```python
from build123d import *
from build123d.topology import SkipClean

# Parameters (mm, degrees)
SKETCH1_R           = 7.5
BOSS_EXTRUDE1_DEPTH = 19
SKETCH1_3_R         = 10
SKETCH1_3_R_2       = 7.5
CUT_EXTRUDE1_DEPTH  = 13
SKETCH2_R           = 6
SKETCH2_R_2         = 5
BOSS_EXTRUDE3_DEPTH = 18
SKETCH11_R          = 10
SKETCH11_R_2        = 7.5
BOSS_EXTRUDE4_DEPTH = 13
SKETCH12_R          = 10
CUT_EXTRUDE7_DEPTH  = 13
SKETCH3_W           = 60
SKETCH3_H           = 5
CUT_EXTRUDE2_DEPTH  = 180
SKETCH4_R           = 7.5
CUT_EXTRUDE3_DEPTH  = 8
SKETCH5_R           = 9
CUT_EXTRUDE4_DEPTH  = 130
SKETCH6_R           = 11
CUT_EXTRUDE5_DEPTH  = 15
SKETCH7_R           = 10
CUT_EXTRUDE6_DEPTH  = 15


with BuildPart() as part:
    # Sketch1 → Boss-Extrude1 (new body)
    with BuildSketch(Plane(origin=(0, 0, 0), x_dir=(1, 0, 0), z_dir=(0, 1, 0))):
        with BuildLine():
            Line((15, 0), (165, 0))
            ThreePointArc((165, 0), (175.606601718, 4.393398282), (180, 15))
            Line((180, 15), (180, 105))
            ThreePointArc((180, 105), (175.606601718, 115.606601718), (165, 120))
            Line((165, 120), (15, 120))
            ThreePointArc((15, 120), (4.393398282, 115.606601718), (0, 105))
            Line((0, 105), (0, 15))
            ThreePointArc((0, 15), (4.393398282, 4.393398282), (15, 0))
        make_face()
        with Locations(Location((15, 15, 0), (0, 0, 270))):
            Circle(SKETCH1_R, mode=Mode.SUBTRACT)
        with Locations(Location((15, 105, 0), (0, 0, 270))):
            Circle(SKETCH1_R, mode=Mode.SUBTRACT)
        with Locations(Location((165, 105, 0), (0, 0, 270))):
            Circle(SKETCH1_R, mode=Mode.SUBTRACT)
        with Locations(Location((165, 15, 0), (0, 0, 270))):
            Circle(SKETCH1_R, mode=Mode.SUBTRACT)
    extrude(amount=BOSS_EXTRUDE1_DEPTH)

    # Sketch1_3 → Cut-Extrude1 (cut)
    # profile 1 of 4: a face of its own
    with BuildSketch(Plane(origin=(0, 0, 0), x_dir=(1, 0, 0), z_dir=(0, 1, 0))):
        with Locations(Location((165, 105, 0), (0, 0, 90))):
            Circle(SKETCH1_3_R)
        with Locations(Location((165, 105, 0), (0, 0, 270))):
            Circle(SKETCH1_3_R_2, mode=Mode.SUBTRACT)
    # profile 2 of 4: a face of its own
    with BuildSketch(Plane(origin=(0, 0, 0), x_dir=(1, 0, 0), z_dir=(0, 1, 0))):
        with Locations(Location((165, 15, 0), (0, 0, 90))):
            Circle(SKETCH1_3_R)
        with Locations(Location((165, 15, 0), (0, 0, 270))):
            Circle(SKETCH1_3_R_2, mode=Mode.SUBTRACT)
    # profile 3 of 4: a face of its own
    with BuildSketch(Plane(origin=(0, 0, 0), x_dir=(1, 0, 0), z_dir=(0, 1, 0))):
        with Locations(Location((15, 105, 0), (0, 0, 90))):
            Circle(SKETCH1_3_R)
        with Locations(Location((15, 105, 0), (0, 0, 270))):
            Circle(SKETCH1_3_R_2, mode=Mode.SUBTRACT)
    # profile 4 of 4: a face of its own
    with BuildSketch(Plane(origin=(0, 0, 0), x_dir=(1, 0, 0), z_dir=(0, 1, 0))):
        with Locations(Location((15, 15, 0), (0, 0, 90))):
            Circle(SKETCH1_3_R)
        with Locations(Location((15, 15, 0), (0, 0, 270))):
            Circle(SKETCH1_3_R_2, mode=Mode.SUBTRACT)
    extrude(amount=CUT_EXTRUDE1_DEPTH, mode=Mode.SUBTRACT)

    # Sketch2 → Boss-Extrude3 (add, symmetric)
    with BuildSketch(Plane.XY.offset(-60)):
        with BuildLine():
            Line((25, 0), (155, 0))
            Line((155, 0), (155, 168))
            ThreePointArc((155, 168), (90, 233), (25, 168))
            Line((25, 168), (25, 0))
        make_face()
        with Locations((90, 218)):
            Circle(SKETCH2_R, mode=Mode.SUBTRACT)
        with Locations((140, 168)):
            Circle(SKETCH2_R, mode=Mode.SUBTRACT)
        with Locations((90, 58)):
            Circle(SKETCH2_R, mode=Mode.SUBTRACT)
        with Locations((40, 168)):
            Circle(SKETCH2_R, mode=Mode.SUBTRACT)
        with Locations((40, 108)):
            Circle(SKETCH2_R, mode=Mode.SUBTRACT)
        with Locations((140, 108)):
            Circle(SKETCH2_R, mode=Mode.SUBTRACT)
        with Locations((54.644660941, 72.644660941)):
            Circle(SKETCH2_R_2, mode=Mode.SUBTRACT)
        with Locations((125.355339059, 203.355339059)):
            Circle(SKETCH2_R_2, mode=Mode.SUBTRACT)
        with BuildLine():
            Line((67.460330813, 141.223829382), (67.460330813, 134.776170618))
            ThreePointArc((67.460330813, 134.776170618), (90, 73), (112.539669187, 134.776170618))
            Line((112.539669187, 134.776170618), (112.539669187, 141.223829382))
            ThreePointArc((112.539669187, 141.223829382), (90, 203), (67.460330813, 141.223829382))
        make_face(mode=Mode.SUBTRACT)
    extrude(amount=BOSS_EXTRUDE3_DEPTH, both=True)

    # Sketch11 → Boss-Extrude4 (add)
    # profile 1 of 4: a face of its own
    with SkipClean():  # the faces are left unmerged after this step: merging them gives an invalid solid
        with BuildSketch(Plane.XZ):
            with Locations((15, -15)):
                Circle(SKETCH11_R)
            with Locations(Location((15, -15, 0), (0, 0, 270))):
                Circle(SKETCH11_R_2, mode=Mode.SUBTRACT)
        # profile 2 of 4: a face of its own
        with BuildSketch(Plane.XZ):
            with Locations((165, -15)):
                Circle(SKETCH11_R)
            with Locations(Location((165, -15, 0), (0, 0, 270))):
                Circle(SKETCH11_R_2, mode=Mode.SUBTRACT)
        # profile 3 of 4: a face of its own
        with BuildSketch(Plane.XZ):
            with Locations((165, -105)):
                Circle(SKETCH11_R)
            with Locations(Location((165, -105, 0), (0, 0, 270))):
                Circle(SKETCH11_R_2, mode=Mode.SUBTRACT)
        # profile 4 of 4: a face of its own
        with BuildSketch(Plane.XZ):
            with Locations((15, -105)):
                Circle(SKETCH11_R)
            with Locations(Location((15, -105, 0), (0, 0, 270))):
                Circle(SKETCH11_R_2, mode=Mode.SUBTRACT)
        extrude(amount=-BOSS_EXTRUDE4_DEPTH)

    # Sketch12 → Cut-Extrude7 (cut)
    with BuildSketch(Plane(origin=(0, 19, 0), x_dir=(1, 0, 0), z_dir=(0, 1, 0))):
        with Locations(Location((15, 105, 0), (0, 0, 270))):
            Circle(SKETCH12_R)
        with Locations(Location((165, 105, 0), (0, 0, 270))):
            Circle(SKETCH12_R)
        with Locations(Location((165, 15, 0), (0, 0, 270))):
            Circle(SKETCH12_R)
        with Locations(Location((15, 15, 0), (0, 0, 270))):
            Circle(SKETCH12_R)
    extrude(amount=-CUT_EXTRUDE7_DEPTH, mode=Mode.SUBTRACT)

    # Sketch3 → Cut-Extrude2 (cut)
    with BuildSketch(Plane(origin=(180, 0, 0), x_dir=(0, 0, -1), z_dir=(1, 0, 0))):
        with Locations((60, 2.5)):
            Rectangle(SKETCH3_W, SKETCH3_H)
    extrude(amount=-CUT_EXTRUDE2_DEPTH, mode=Mode.SUBTRACT)

    # Sketch4 → Cut-Extrude3 (cut)
    with BuildSketch(Plane(origin=(0, 0, -78), x_dir=(-1, 0, 0), z_dir=(0, 0, -1))):
        with Locations((-90, 218)):
            Circle(SKETCH4_R)
        with Locations((-40, 168)):
            Circle(SKETCH4_R)
        with Locations((-40, 108)):
            Circle(SKETCH4_R)
        with Locations((-90, 58)):
            Circle(SKETCH4_R)
        with Locations((-140, 108)):
            Circle(SKETCH4_R)
        with Locations((-140, 168)):
            Circle(SKETCH4_R)
    cut_extrude3 = extrude(amount=-CUT_EXTRUDE3_DEPTH, mode=Mode.SUBTRACT)

    # Mirror1: Cut-Extrude3 across plane
    add(cut_extrude3.mirror(Plane.XY.offset(-60)), mode=Mode.SUBTRACT)

    # Sketch5 → Cut-Extrude4 (cut)
    with BuildSketch(Plane.ZY.offset(-25)):
        with Locations((-60, 138)):
            Circle(SKETCH5_R)
    extrude(amount=-CUT_EXTRUDE4_DEPTH, mode=Mode.SUBTRACT)

    # Sketch6 → Cut-Extrude5 (cut)
    with BuildSketch(Plane.ZY.offset(-25)):
        with Locations((-60, 138)):
            Circle(SKETCH6_R)
    extrude(amount=-CUT_EXTRUDE5_DEPTH, mode=Mode.SUBTRACT)

    # Sketch7 → Cut-Extrude6 (cut)
    with BuildSketch(Plane(origin=(155, 0, 0), x_dir=(0, 0, -1), z_dir=(1, 0, 0))):
        with Locations((60, 138)):
            Circle(SKETCH7_R)
    extrude(amount=-CUT_EXTRUDE6_DEPTH, mode=Mode.SUBTRACT)


solid = part.part
```
Input: part model. Units: mm. Frame: model coordinates. A direction names the side the tool comes from. Give positions to 0.01 mm unless a question says otherwise; leave off trailing zeros. Loops run counter-clockwise (first coordinate to the right, second up) from the corner with the lowest first, then second, coordinate; pieces in that order, holes last. Notation, with made-up numbers: (-8, 67.5) -> (36, 67.5) arc R24 cw to (36, 78.5) -> close; hole circle Ø11 at (-32.75, 14.25). An arc over 180 degrees is marked (long way). Use a Markdown table: item, result.
Q1. Access query for faces 1 (the flat face through (88, 224, -50)), 2 (the cylindrical face through (40.976, 175.436, -74.056)), 3 (the cylindrical face through (155.24, 12.59, -17.17)), 4 (the flat face through (112.54, 138, -73)), 5 (the flat face through (91, 5, -60)). Directions: +Z, -Z, +X, -X, +Y, -Y. A direction counts if a zero-diameter tool reaches every point of the face in a straight line with its end or side. Return the directions, or none.
Entries:
| item | result |
|---|---|
| face 1 | +Z |
| face 2 | -Z |
| face 3 | +Y |
| face 4 | +Z, -Z |
| face 5 | +X, -X, -Y |
Q2. Section query A-A, the plane y = 58. Return the cut outline in (x, z).
Entries:
| item | result |
|---|---|
| outline | (25, -78) -> (82.5, -78) -> (82.5, -70) -> (84, -70) -> (84, -50) -> (82.5, -50) -> (82.5, -42) -> (25, -42) -> close; (96, -70) -> (97.5, -70) -> (97.5, -78) -> (155, -78) -> (155, -42) -> (97.5, -42) -> (97.5, -50) -> (96, -50) -> close |
Q3. Section query D-D, the plane z = -84. Return the cut outline in (x, y).
Entries:
| item | result |
|---|---|
| outline | (0, 5) -> (180, 5) -> (180, 19) -> (0, 19) -> close |
Q4. First-contact query: P1, Ø1.5, axis at x = 115.5, z = -98.5, coming from the +Y side; P2, Ø1.9, axis at y = 137, z = -72, coming from the -X side; P3, Ø13.5, axis at x = 40, y = 168, coming from the -Z side. Flat tips, straight axial feed; report the tip coordinate or a pass-through.
Entries:
| item | result |
|---|---|
| P1 | stops at y = 19 |
| P2 | stops at x = 25 |
| P3 | stops at z = -70 |
Q5. Section query C-C, the plane y = 89.5. Return the cut outline in (x, z).
Entries:
| item | result |
|---|---|
| outline | (25, -78) -> (60.29, -78) -> (60.29, -42) -> (25, -42) -> close; (119.71, -78) -> (155, -78) -> (155, -42) -> (119.71, -42) -> close |
Q6. Section query B-B, the plane x = 90. State how many separate pieces and enclosed holes the cut face has, plus the area to 3 significant figures.
Entries:
| item | result |
|---|---|
| separate pieces | 4 |
| enclosed holes | 0 |
| area | 4,040 mm² |
Q7. Ray query, probe 1 along X at (y, z) = (9, -105); probe 2 along Y at (x, z) = (90, -63); probe 3 along Z at (x, y) = (125, 138). Return the intervals inside material, ascending. Write a range as from..to.
Entries:
| item | result |
|---|---|
| probe 1 | x = 0..5, 25..155, 175..180 |
| probe 2 | y = 5..52, 64..73, 203..212, 224..233 |
| probe 3 | z = -78..-69, -51..-42 |
Q8. Pull-direction query (Z, two-part tool) for faces 6 (the cylindrical face through (175.49, 9.37, -4.28)), 7 (the cylindrical face through (155.24, 12.59, -107.17)), 8 (the cylindrical face through (135.968, 174.324, -45.944)); classes: pulls with the +Z half, pulls with the -Z half, needs draft (parallel to the pull), parting line crosses it, or undercut.
Entries:
| item | result |
|---|---|
| face 6 | pulls with the +Z half |
| face 7 | undercut |
| face 8 | needs draft |
